Can you work these out from the model? Positions are in its coordinate system, mm. Give positions to 0.01 mm unless a question says otherwise; leave off trailing zeros. Loops run counter-clockwise (first coordinate to the right, second up) from the corner with the lowest first, then second, coordinate; pieces in that order, holes last. Notation, with made-up numbers: M 33.5,-24 L 86.5,-24 A19 ccw 86.5,12 Z; hole C 53.5,35 d6. An arc over 180 degrees is marked long. Use CSV: the item, a comma, the result in double quotes.
Autodesk Inventor part; units mm, degrees
ref_plane "YZ Plane" through (0, 0, 0) normal (1, 0, 0) x (0, 1, 0)
ref_plane "XZ Plane" through (0, 0, 0) normal (0, 1, 0) x (-1, 0, 0)
ref_plane "XY Plane" through (0, 0, 0) normal (0, 0, 1) x (1, 0, 0)
sketch "Skizze3" plane through (0, 0, 0) normal (0, 0, 1) x (1, 0, 0)
  line L0 (0, 0) -> (7, 0)
  line L1 (7, 0) -> (7, 7)
  line L2 (7, 7) -> (0, 7)
  line L3 (0, 7) -> (0, 0)
  point P0 (3.5, 3.5)
  point P1 (3.5, 7)
  point P2 (0, 3.5)
  dimension "d4" = 7
  dimension "d5" = 7
extrude "Extrusion3" add sketch "Skizze3" along normal blind 2.2
fillet "Rundung1" radius 1 4 edges at (7, 7, 1.1) (0, 7, 1.1) (0, 0, 1.1) (7, 0, 1.1)
hole "Bohrung1" at (3.5, 3.5, 0) direction (0, 0, 1) diameter 3.242 depth 11.8
equation "\"d5\" = d4"
properties part number "BT004_trajan20_22"
Q1. I want a section at A-A, the plane x = 3.5. Please give me the cut outline in (y, z), then the cut area to 3 significant figures.
Model answer:
outline,"M 0,0 L 1.88,0 L 1.88,2.2 L 0,2.2 Z; M 5.12,0 L 7,0 L 7,2.2 L 5.12,2.2 Z"
area,"8.27 mm2"
Q2. Please list where these lines run through material, in increasing order: L1, parallel to Y at x = 3.5, z = 1.6; L2, parallel to X at y = 2.5, z = 1.65. Write a range as from..to.
Model answer:
L1,"0..1.88, 5.12..7"
L2,"0..2.22, 4.78..7"
Q3. I want a section at C-C, the plane z = 0.85. Please give me the cut outline in (x, y).
Model answer:
outline,"M 0,1 A1 ccw 1,0 L 6,0 A1 ccw 7,1 L 7,6 A1 ccw 6,7 L 1,7 A1 ccw 0,6 Z; hole C 3.5,3.5 d3.24"
Q4. I'm going to push a flat-ended pin straight in: P1, Ø4, axis at x = 3.5, y = 3.5, coming from the +Z side. Where does the tip first touch, or does it pass through?
Model answer:
P1,"z = 2.2"
Q5. I want a section at B-B, the plane y = 4.75. Please give me the cut outline in (x, z), then the cut area to 3 significant figures.
Model answer:
outline,"M 0,0 L 2.47,0 L 2.47,2.2 L 0,2.2 Z; M 4.53,0 L 7,0 L 7,2.2 L 4.53,2.2 Z"
area,"10.9 mm2"
Q6. I want a section at D-D, the plane x = 6.5. Please give me the cut outline in (y, z).
Model answer:
outline,"M 0.13,0 L 6.87,0 L 6.87,2.2 L 0.13,2.2 Z"
Q7. If we mould it in two halves opening along Y, with no side actions, what happens to faces 1 (the flat face through (7, 3, 1)), 2 (the cylindrical face through (6.699, 0.285, 1.115)), 3 (the cylindrical face through (5.082, 3.149, 1.115))? For each: released by +Y, released by -Y, zero draft, split by the parting line, or undercut.
Model answer:
face 1,"zero draft"
face 2,"released by -Y"
face 3,"undercut"
